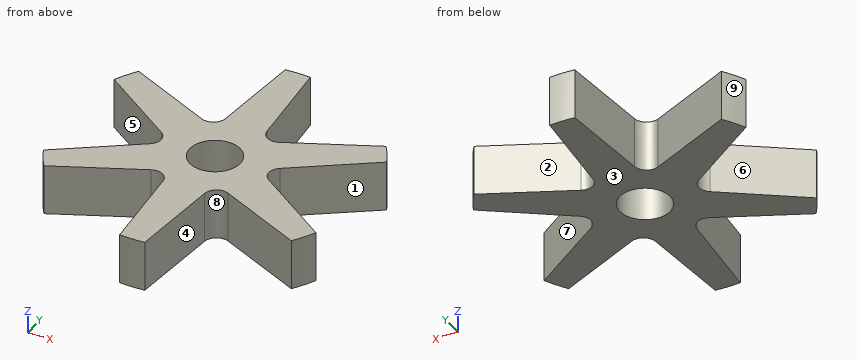
Autodesk Inventor part; units mm, degrees
ref_plane "YZ Plane" through (0, 0, 0) normal (1, 0, 0) x (0, 1, 0)
ref_plane "XZ Plane" through (0, 0, 0) normal (0, 1, 0) x (-1, 0, 0)
ref_plane "XY Plane" through (0, 0, 0) normal (0, 0, 1) x (1, 0, 0)
sketch "Sketch1" plane through (0, 0, 0) normal (0, 0, 1) x (1, 0, 0)
  arc A0 (3.175, 37.9675) -> (-3.175, 37.9675) centre (0, 0) ccw
  line L0 (-3.175, 37.9675) -> (-5.6418, 9.7719)
  line L1 (0, 38.1) -> (0, 0) construction
  arc A1 (-3.175, 37.9675) -> (-31.2933, 21.7334) centre (0, 0) ccw construction
  line L2 (-5.6418, 9.7719) -> (5.6418, 9.7719) construction
  line L3 (5.6418, 9.7719) -> (11.2836, 0) construction
  line L4 (11.2836, 0) -> (5.6418, -9.7719) construction
  line L5 (5.6418, -9.7719) -> (-5.6418, -9.7719) construction
  line L6 (-5.6418, -9.7719) -> (-11.2836, 0) construction
  line L7 (-11.2836, 0) -> (-5.6418, 9.7719) construction
  line L8 (3.175, 37.9675) -> (5.6418, 9.7719)
  line L9 (0, 0) -> (-32.9956, 19.05) construction
  line L10 (0, 0) -> (32.9956, 19.05) construction
  line L11 (0, 0) -> (-32.9956, -19.05) construction
  line L12 (0, 0) -> (32.9956, -19.05) construction
  line L13 (0, 0) -> (0, -38.1) construction
  line L14 (5.6418, 9.7719) -> (31.2933, 21.7334)
  line L15 (11.2836, 0) -> (34.4683, 16.2341)
  line L16 (11.2836, 0) -> (34.4683, -16.2341)
  line L17 (5.6418, -9.7719) -> (31.2933, -21.7334)
  arc A2 (31.2933, 21.7334) -> (3.175, 37.9675) centre (0, 0) ccw construction
  arc A3 (34.4683, 16.2341) -> (31.2933, 21.7334) centre (0, 0) ccw
  arc A4 (34.4683, -16.2341) -> (34.4683, 16.2341) centre (0, 0) ccw construction
  arc A5 (31.2933, -21.7334) -> (34.4683, -16.2341) centre (0, 0) ccw
  line L18 (5.6418, -9.7719) -> (3.175, -37.9675)
  line L19 (-5.6418, -9.7719) -> (-3.175, -37.9675)
  line L20 (-5.6418, -9.7719) -> (-31.2933, -21.7334)
  line L21 (-11.2836, 0) -> (-34.4683, -16.2341)
  line L22 (-11.2836, 0) -> (-34.4683, 16.2341)
  line L23 (-5.6418, 9.7719) -> (-31.2933, 21.7334)
  arc A6 (-31.2933, 21.7334) -> (-34.4683, 16.2341) centre (0, 0) ccw
  arc A7 (-34.4683, 16.2341) -> (-34.4683, -16.2341) centre (0, 0) ccw construction
  arc A8 (-34.4683, -16.2341) -> (-31.2933, -21.7334) centre (0, 0) ccw
  arc A9 (-31.2933, -21.7334) -> (-3.175, -37.9675) centre (0, 0) ccw construction
  arc A10 (-3.175, -37.9675) -> (3.175, -37.9675) centre (0, 0) ccw
  arc A11 (3.175, -37.9675) -> (31.2933, -21.7334) centre (0, 0) ccw construction
  circle A12 centre (0, 0) radius 6.35
  dimension "d10" = 38.1
  dimension "d1" = 6.35
  dimension "d2" = 3.175
  dimension "d3" = 5
  dimension "d5" = 5
  dimension "d6" = 5
  dimension "d7" = 5
  dimension "d8" = 5
  dimension "d9" = 5
  dimension "d13" = 12.7
extrude "Extrusion1" add sketch "Sketch1" along normal blind 12.7
fillet "Fillet1" radius 3.175 6 edges at (5.6418, 9.7719, 6.35) (-5.6418, 9.7719, 6.35) (-11.2836, 0, 6.35) (-5.6418, -9.7719, 6.35) (5.6418, -9.7719, 6.35) (11.2836, 0, 6.35)
equation "\"d2\" = 0.5 * d1"
equation "\"d5\" = d3"
equation "\"d6\" = d3"
equation "\"d8\" = d6"
equation "\"d9\" = d8"
properties part number "rubber intake star"
Read the model definition and answer for the solid it produces. Units are mm, in the model's axes. Face numbers are marked on the shaded views. A direction names the side the tool comes from. Give positions to 0.01 mm unless a question says otherwise; leave off trailing zeros. Order: outer loops, then holes, each group sorted by start corner. A loop starts at its lowest first (then second) coordinate and runs counter-clockwise, first axis right, second up.
(1) Find section A-A (x = 0). Give the vertices of the cut face in (y, z).
(2) For the marked faces 1, 2, 3, 4 and 5, determine the directions among +Z, -Z, +X, -X, +Y, -Y from which every point of the face is accessible in a straight line to the end or side of a thin tool.
(3) Straight lines are drawn through the part: L1, parallel to X at y = 4, z = 7; L2, parallel to Y at x = -19.5, z = 9; L3, parallel to X at y = 14, z = 9.75. For each, find the intervals that lie inside material, in ascending order.
(4) For a pull along Y with two mould halves and no side action, classify the marked faces 6, 7, 8 and 9 as released by +Y, released by -Y, zero draft, split by the parting line, or undercut.
(5) Find section B-B (y = 0). Give the vertices of the cut face in (x, z), plus the area to 3 significant figures.
(6) Find section D-D (y = -19.5). Give the vertices of the cut face in (x, z).
(7) Given pin 1 (2 mm diameter, centred on x = 26, z = 3.5, fed in from -Y); pin 2 (3 mm diameter, centred on x = -21.5, z = 5, fed in from +Y); pin 3 (1 mm diameter, centred on x = -20.5, z = 8, fed in from +Y), each flat-ended and moving along its own axis, determine where each tip first touches the part or whether it passes through.
Result sheet:
1. outline: (-38.1, 0) - (-6.35, 0) - (-6.35, 12.7) - (-38.1, 12.7) - close; (6.35, 0) - (38.1, 0) - (38.1, 12.7) - (6.35, 12.7) - close
2. face 1: +Z, -Z, +X
2. face 2: +Z, -Z, +Y
2. face 3: -Z, +X, -X, +Y, -Y
2. face 4: +Z, -Z, -Y
2. face 5: +Z, -Z, -X
3. L1: x = -17 to -4.93, 4.93 to 17
3. L2: y = -16.23 to -5.75, 5.75 to 16.23
3. L3: x = -31.28 to -14.71, -5.29 to 5.29, 14.71 to 31.28
4. face 6: undercut
4. face 7: undercut
4. face 8: released by -Y
4. face 9: released by +Y
5. outline: (-13.64, 0) - (-6.35, 0) - (-6.35, 12.7) - (-13.64, 12.7) - close; (6.35, 0) - (13.64, 0) - (13.64, 12.7) - (6.35, 12.7) - close
5. area: 185 mm2
6. outline: (-32.73, 0) - (-26.5, 0) - (-26.5, 12.7) - (-32.73, 12.7) - close; (-4.79, 0) - (4.79, 0) - (4.79, 12.7) - (-4.79, 12.7) - close; (26.5, 0) - (32.73, 0) - (32.73, 12.7) - (26.5, 12.7) - close
7. pin 1: stops at y = -19.73
7. pin 2: stops at y = 17.87
7. pin 3: stops at y = 16.93
